Answer from the drawing. Dimensions are ordinates in mm from the lowest x, y and z of the part. Coordinates: 2 decimals unless noted, no trailing zeros. Write each loop counter-clockwise with the first axis right and the second up, starting at its lowest first coordinate (ties: lowest second). Pieces come first, ordered by that corner, then holes.
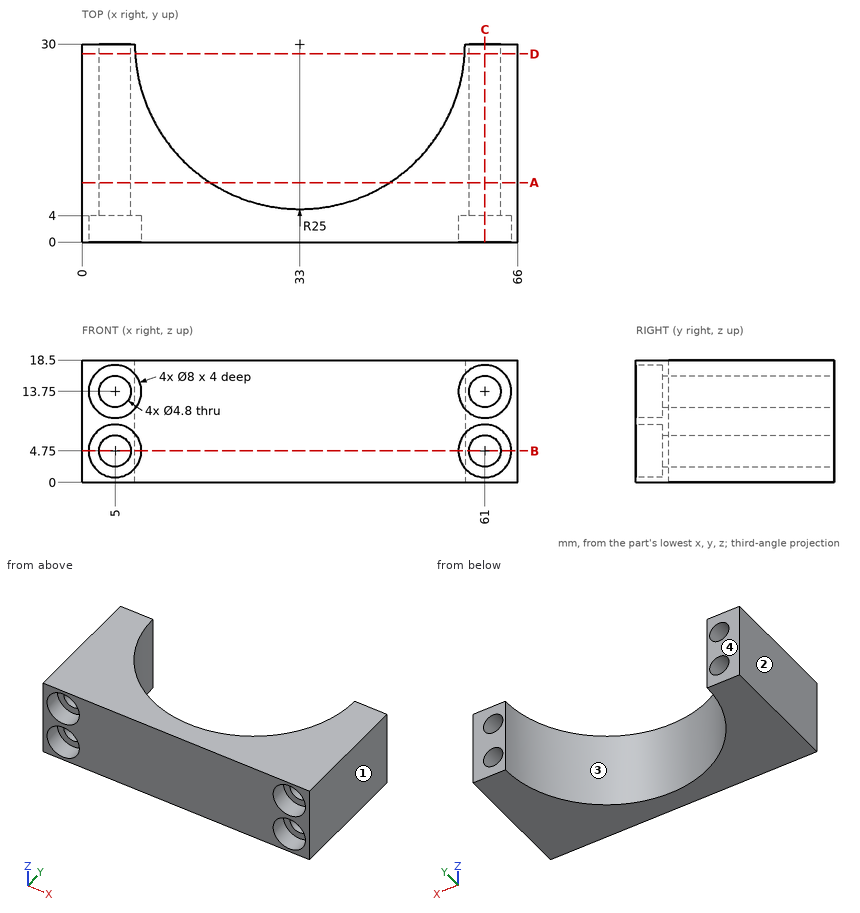
(1) Section C-C, the plane x = 61 is taken. Write down the section's boundary in (y, z).
(2) Find the intervals of material crossed by probe 1 along Z at (x, y) = (5, 18.25); probe 2 along Z at (x, y) = (61, 1.4); probe 3 along X at (y, z) = (3, 7.5), in increasing order.
(3) Each of these flat-tipped pins is pushed along its axis until it touches: pin 1 (4 mm diameter, centred on x = 35.5, z = 5, fed in from +Y); pin 2 (5.5 mm diameter, centred on x = 5, z = 13.75, fed in from -Y); pin 3 (1 mm diameter, centred on x = 14, z = 15, fed in from +Y). Where does it stop, or does it pass through?
(4) For a pull along X with two mould halves and no side action, classify the marked faces 1, 2, 3 and 4 as pulls with the +X half, pulls with the -X half, needs draft (parallel to the pull), parting line crosses it, or undercut.
(5) Section D-D, the plane y = 28.5 is taken. Write down the section's boundary in (x, z).
(6) Section B-B, the plane z = 4.75 is taken. Write down the section's boundary in (x, y), plus the area to 3 significant figures.
(7) Section A-A, the plane y = 9 is taken. Write down the section's boundary in (x, z), plus the area to 3 significant figures.
Solution:
1. outline: (0, 0) - (30, 0) - (30, 2.35) - (4, 2.35) - (4, 0.75) - (0, 0.75) - close; (0, 8.75) - (4, 8.75) - (4, 7.15) - (30, 7.15) - (30, 11.35) - (4, 11.35) - (4, 9.75) - (0, 9.75) - close; (0, 17.75) - (4, 17.75) - (4, 16.15) - (30, 16.15) - (30, 18.5) - (0, 18.5) - close
2. probe 1: z = 0 to 2.35, 7.15 to 11.35, 16.15 to 18.5
2. probe 2: z = 0 to 0.75, 8.75 to 9.75, 17.75 to 18.5
2. probe 3: x = 0 to 2.1, 7.9 to 58.1, 63.9 to 66
3. pin 1: stops at y = 5.41
3. pin 2: stops at y = 4
3. pin 3: stops at y = 14.36
4. face 1: pulls with the +X half
4. face 2: pulls with the -X half
4. face 3: undercut
4. face 4: needs draft
5. outline: (0, 0) - (8.05, 0) - (8.05, 18.5) - (0, 18.5) - close; (57.95, 0) - (66, 0) - (66, 18.5) - (57.95, 18.5) - close; hole circle Ø4.8 at (5, 4.75); hole circle Ø4.8 at (5, 13.75); hole circle Ø4.8 at (61, 4.75); hole circle Ø4.8 at (61, 13.75)
6. outline: (0, 0) - (1, 0) - (1, 4) - (2.6, 4) - (2.6, 30) - (0, 30) - close; (7.4, 4) - (9, 4) - (9, 0) - (57, 0) - (57, 4) - (58.6, 4) - (58.6, 30) - (58, 30) arc R25 cw to (8, 30) - (7.4, 30) - close; (63.4, 4) - (65, 4) - (65, 0) - (66, 0) - (66, 30) - (63.4, 30) - close
6. area: 685 mm2
7. outline: (0, 0) - (19.44, 0) - (19.44, 18.5) - (0, 18.5) - close; (46.56, 0) - (66, 0) - (66, 18.5) - (46.56, 18.5) - close; hole circle Ø4.8 at (5, 4.75); hole circle Ø4.8 at (5, 13.75); hole circle Ø4.8 at (61, 4.75); hole circle Ø4.8 at (61, 13.75)
7. area: 647 mm2
